The listing builds one solid part. Answer for the finished solid, in the listing's coordinates (mm). Face numbers are marked on the shaded views. Give positions to 0.01 mm unless a question says otherwise; leave off trailing zeros. Order: outer loops, then holes, each group sorted by start corner. A loop starts at its lowest first (then second) coordinate and runs counter-clockwise, first axis right, second up. Notation, with made-up numbers: (46.5, 77) -> (100.5, 77) arc R26 cw to (100.5, 98) -> close; hole circle Ø11 at (-32, 64). An arc over 180 degrees is marked (long way). Write item = value, one per line. Start each with the question number.
Autodesk Inventor part; units mm, degrees
ref_plane "YZ Plane" through (0, 0, 0) normal (1, 0, 0) x (0, 1, 0)
ref_plane "XZ Plane" through (0, 0, 0) normal (0, 1, 0) x (-1, 0, 0)
ref_plane "XY Plane" through (0, 0, 0) normal (0, 0, 1) x (1, 0, 0)
sketch "Sketch1" plane through (0, 0, 0) normal (0, 0, 1) x (1, 0, 0)
  line L0 (0, 0) -> (51.5, 0)
  line L1 (51.5, 0) -> (51.5, 30)
  line L2 (51.5, 30) -> (0, 30)
  line L3 (0, 30) -> (0, 0)
  dimension "d0" = 51.5
  dimension "d1" = 30
extrude "Extrusion1" add sketch "Sketch1" along normal blind 2.9
sketch "Sketch2" plane through (0, 0, 0) normal (0, -1, 0) x (1, 0, 0)
  line L0 (0, 0) -> (0, 2.9)
  line L1 (0, 2.9) -> (3, 2.9)
  line L2 (51.5, 2.9) -> (0, 2.9)
  line L3 (51.5, 0) -> (0, 0)
  line L4 (3, 2.9) -> (0, 0)
  line L5 (51.5, 2.9) -> (48.5, 2.9)
  line L6 (48.5, 2.9) -> (51.5, 0)
  line L7 (3, 2.9) -> (3, 0)
  line L8 (3, 0) -> (48, 0)
  line L9 (48, 0) -> (48, 1.9)
  line L10 (48, 1.9) -> (3, 1.9)
  line L11 (3, 1.9) -> (3, 0)
  line L12 (51.5, 2.9) -> (51.5, 0)
  dimension "d4" = 3
  dimension "d5" = 3
  dimension "d6" = 1.9
extrude "Extrusion2" cut sketch "Sketch2" against normal through all contours L0 L1 L4 | L7 L10 L9 L3 | L2 L12 L6
fillet "Fillet1" radius 0.3 4 edges at (3, 15, 2.9) (0, 15, 0) (48.5, 15, 2.9) (51.5, 15, 0)
sketch "Sketch4" plane through (48, 0, 1.9) normal (0, 0, -1) x (-1, 0, 0)
  line L0 (45, 0) -> (0, 0)
  line L1 (45, 0) -> (40, 0)
  line L2 (40, 0) -> (40, 5)
  circle A0 centre (40, 5) radius 2
  circle A1 centre (31.5, 5) radius 2
  circle A2 centre (23, 5) radius 2
  circle A3 centre (14.5, 5) radius 2
  circle A4 centre (6, 5) radius 2
  circle A5 centre (40, 11.5) radius 2
  circle A6 centre (31.5, 11.5) radius 2
  circle A7 centre (23, 11.5) radius 2
  circle A8 centre (14.5, 11.5) radius 2
  circle A9 centre (6, 11.5) radius 2
  circle A10 centre (40, 18) radius 2
  circle A11 centre (31.5, 18) radius 2
  circle A12 centre (23, 18) radius 2
  circle A13 centre (14.5, 18) radius 2
  circle A14 centre (6, 18) radius 2
  circle A15 centre (40, 24.5) radius 2
  circle A16 centre (31.5, 24.5) radius 2
  circle A17 centre (23, 24.5) radius 2
  circle A18 centre (14.5, 24.5) radius 2
  circle A19 centre (6, 24.5) radius 2
  point P0 (48, 0)
  dimension "d10" = 5
  dimension "d11" = 5
  dimension "d12" = 4
  dimension "d15" = 8.5
  dimension "d18" = 6.5
extrude "Extrusion3" cut sketch "Sketch4" against normal blind 2.9
properties part number "PalmSupport"
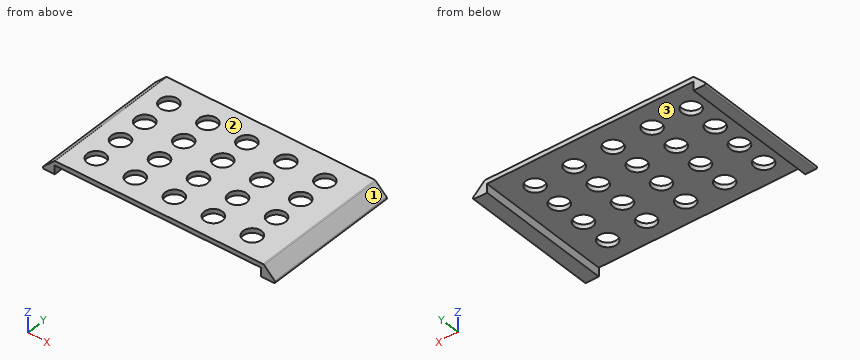
Item 1: Consider L1, parallel to Y at x = 42, z = 2.45; L2, parallel to Z at x = 29.5, y = 21.75; L3, parallel to X at y = 8.5, z = 1.05. Determine where each line is inside the solid, lowest interval first. Write a range as from..to.
Item 2: A cutting plane is placed at D-D, the plane x = 43. Write down the section's boundary in (y, z).
Item 3: A cutting plane is placed at A-A, the plane x = 8. Write down the section's boundary in (y, z).
Item 4: A cutting plane is placed at C-C, the plane z = 1.4. Write down the section's boundary in (x, y), plus the area to 3 significant figures.
Item 5: A cutting plane is placed at B-B, the plane y = 5. Count the separate pieces of the cut face and the enclosed holes in it, plus the area to 3 significant figures.
Item 6: The mould has two halves that part along X. Classify the marked faces 1, 2 and 3: +X half, -X half, draft (parallel to the pull), parting line (faces both ways), or undercut.
Item 7: Flat-ended cylindrical pins translate along their axes: pin 1 (6.5 mm diameter, centred on x = 8, y = 11.5, fed in from -Z); pin 2 (1.5 mm diameter, centred on y = 16, z = 2, fed in from -X); pin 3 (4.5 mm diameter, centred on x = 16.5, y = 11.5, fed in from +Z). Find the tip coordinate at first contact, or state that the pin passes through.
Check values:
q1.L1 = 0..3, 7..9.5, 13.5..16, 20..22.5, 26.5..30
q1.L2 = 1.9..2.9
q1.L3 = 1.09..3, 48..50.41
q2.outline = (0, 1.9) -> (3.27, 1.9) -> (3.27, 2.9) -> (0, 2.9) -> close; (6.73, 1.9) -> (9.77, 1.9) -> (9.77, 2.9) -> (6.73, 2.9) -> close; (13.23, 1.9) -> (16.27, 1.9) -> (16.27, 2.9) -> (13.23, 2.9) -> close; (19.73, 1.9) -> (22.77, 1.9) -> (22.77, 2.9) -> (19.73, 2.9) -> close; (26.23, 1.9) -> (30, 1.9) -> (30, 2.9) -> (26.23, 2.9) -> close
q3.outline = (0, 1.9) -> (3, 1.9) -> (3, 2.9) -> (0, 2.9) -> close; (7, 1.9) -> (9.5, 1.9) -> (9.5, 2.9) -> (7, 2.9) -> close; (13.5, 1.9) -> (16, 1.9) -> (16, 2.9) -> (13.5, 2.9) -> close; (20, 1.9) -> (22.5, 1.9) -> (22.5, 2.9) -> (20, 2.9) -> close; (26.5, 1.9) -> (30, 1.9) -> (30, 2.9) -> (26.5, 2.9) -> close
q4.outline = (1.45, 0) -> (3, 0) -> (3, 30) -> (1.45, 30) -> close; (48, 0) -> (50.05, 0) -> (50.05, 30) -> (48, 30) -> close
q4.area = 108 mm^2
q5.separate_pieces = 6
q5.enclosed_holes = 0
q5.area = 34.9 mm^2
q6.face_1 = +X half
q6.face_2 = draft
q6.face_3 = undercut
q7.pin_1 = 1.9
q7.pin_2 = 1.29
q7.pin_3 = 2.9
